Input: part model. Units: mm. Frame: model coordinates. A direction names the side the tool comes from. Coordinates: 2 decimals unless noted, no trailing zeros. Order: outer loops, then holes, each group sorted by start corner. A loop starts at its lowest first (then second) coordinate and runs counter-clockwise, first axis right, second up.
from build123d import *

# Parameters (mm, degrees)
ESQUISSE1_R             = 26.25
BOSS_EXTRU_1_DEPTH      = 5
ESQUISSE2_R             = 1.5
ENL_V_MAT_EXTRU_1_DEPTH = 5
ENL_V_START             = -5
ESQUISSE3_R             = 26.25
ESQUISSE3_R_2           = 2
ENL_V_MAT_EXTRU_2_DEPTH = 5
CONG_1_R                = 2
ESQUISSE4_R             = 1.125
ENL_V_MAT_EXTRU_3_DEPTH = 10
ESQUISSE5_R             = 4
ESQUISSE5_R_2           = 2
BOSS_EXTRU_2_DEPTH      = 3


with BuildPart() as part:
    # Esquisse1 → Boss.-Extru.1 (new body)
    with BuildSketch(Plane.XY):
        Circle(ESQUISSE1_R)
    extrude(amount=BOSS_EXTRU_1_DEPTH)

    # Esquisse2 → Enlèv. mat.-Extru.1 (cut)
    with BuildSketch(Plane.XY.offset(5)):
        Circle(ESQUISSE2_R)
    extrude(amount=-ENL_V_MAT_EXTRU_1_DEPTH, mode=Mode.SUBTRACT)

    # Esquisse3 → Enlèv. mat.-Extru.2 (cut)
    # profile 1 of 2: a face of its own
    with BuildSketch(Plane.XY.offset(5).offset(ENL_V_START)):
        Circle(ESQUISSE3_R)
        with BuildLine():
            Line((9, -2.5), (4, -2.5))
            Line((4, -2.5), (4, -19.5))
            ThreePointArc((4, -19.5), (0, -23.5), (-4, -19.5))
            Line((-4, -19.5), (-4, -2.5))
            Line((-4, -2.5), (-9, -2.5))
            ThreePointArc((-9, -2.5), (-11.5, 0), (-9, 2.5))
            Line((-9, 2.5), (-3.122498999, 2.5))
            ThreePointArc((-3.122498999, 2.5), (-2.828427125, 2.828427125), (-2.5, 3.122498999))
            Line((-2.5, 3.122498999), (-2.5, 9))
            ThreePointArc((-2.5, 9), (0, 11.5), (2.5, 9))
            Line((2.5, 9), (2.5, 3.122498999))
            ThreePointArc((2.5, 3.122498999), (2.828427125, 2.828427125), (3.122498999, 2.5))
            Line((3.122498999, 2.5), (9, 2.5))
            ThreePointArc((9, 2.5), (11.5, 0), (9, -2.5))
        make_face(mode=Mode.SUBTRACT)
    # profile 2 of 2: a face of its own
    with BuildSketch(Plane.XY.offset(5).offset(ENL_V_START)):
        with Locations((0, -19.5)):
            Circle(ESQUISSE3_R_2)
    extrude(amount=ENL_V_MAT_EXTRU_2_DEPTH, mode=Mode.SUBTRACT)

    # Congé1
    # the kernel refuses this fillet: 2 mm, written as the material it adds along each edge
    with BuildSketch(Plane(origin=(-4, -2.5, 0), x_dir=(0, -1, 0), z_dir=(0, 0, 1)), Plane(origin=(4, -2.5, 0), x_dir=(1, 0, 0), z_dir=(0, 0, 1))) as cong_1_piece_1:
        with BuildLine():
            CenterArc((CONG_1_R, -CONG_1_R), CONG_1_R, 90, 90)
            Line((0, -CONG_1_R), (0, 0))
            Line((0, 0), (CONG_1_R, 0))
        make_face()
    extrude(amount=5)
    with BuildSketch(Plane(origin=(-3.122498999, 2.5, 0), x_dir=(-1, 0, 0), z_dir=(0, 0, 1))) as cong_1_piece_2:
        with BuildLine():
            CenterArc((0.846127967, -2), CONG_1_R, 90, 41.409622109)
            ThreePointArc((-0.476747688, -0.5), (-0.227558946, -0.260311955), (0, 0))
            Line((0, 0), (0.846127967, 0))
        make_face()
    extrude(amount=5)
    with BuildSketch(Plane(origin=(-2.5, 3.122498999, 0), x_dir=(-0.7237350132500174, -0.6900779887780779, 0), z_dir=(0, 0, 1)), Plane(origin=(3.122498999, 2.5, 0), x_dir=(-0.6900779887780603, 0.7237350132500343, 0), z_dir=(0, 0, 1))) as cong_1_piece_3:
        with BuildLine():
            CenterArc((0.863575741, -1.992528413), CONG_1_R, 94.954095219, 41.409622109)
            Line((-0.583894286, -0.612372436), (0, 0))
            ThreePointArc((0, 0), (0.345430296, -0.014943173), (0.690860592, 0))
        make_face()
    extrude(amount=5)
    with BuildSketch(Plane(origin=(2.5, 3.122498999, 0), x_dir=(0.7237350132500171, -0.6900779887780782, 0), z_dir=(0, 0, 1))) as cong_1_piece_4:
        with BuildLine():
            CenterArc((0.863575741, 1.992528413), CONG_1_R, 223.636282672, 41.409622109)
            Line((-0.583894286, 0.612372436), (0, 0))
            ThreePointArc((0, 0), (0.345430296, 0.014943173), (0.690860592, 0))
        make_face()
    extrude(amount=5)

    # Esquisse4 → Enlèv. mat.-Extru.3 (cut)
    with BuildSketch(Plane.XY.offset(5)):
        with Locations((8, 0)):
            Circle(ESQUISSE4_R)
        with Locations((-8, 0)):
            Circle(ESQUISSE4_R)
        with Locations((0, 8)):
            Circle(ESQUISSE4_R)
    extrude(amount=-ENL_V_MAT_EXTRU_3_DEPTH, mode=Mode.SUBTRACT)

    # Esquisse5 → Boss.-Extru.2 (add)
    with BuildSketch(Plane.XY.offset(5)):
        with Locations((0, -19.5)):
            Circle(ESQUISSE5_R)
        with Locations((0, -19.5)):
            Circle(ESQUISSE5_R_2, mode=Mode.SUBTRACT)
    extrude(amount=BOSS_EXTRU_2_DEPTH)


solid = part.part
Item 1: Cut plane C-C on x = 8. Return loops of the section in (y, z) (3 decimals).
Response values:
outline: (-2.5, 0) - (-1.125, 0) - (-1.125, 5) - (-2.5, 5) - close; (1.125, 0) - (2.5, 0) - (2.5, 5) - (1.125, 5) - close
Item 2: Ray query, probe 1 along Y at (x, z) = (0, 2.6) (3 decimals); probe 2 along Y at (x, z) = (8, 3.1) (3 decimals); probe 3 along Z at (x, y) = (2, 4). Return the intervals inside material, ascending.
Response values:
probe 1: y = -23.5 to -21.5, -17.5 to -1.5, 1.5 to 6.875, 9.125 to 11.5
probe 2: y = -2.5 to -1.125, 1.125 to 2.5
probe 3: z = 0 to 5
Item 3: Access query for faces 4 (the face through (-7, 2.5, 2)), 5 (the face through (-4.57, -3.1, 2.46)), 6 (the face through (-0.24, 6.9, 2.54)), 7 (the face through (6, 2.5, 2)), 8 (the face through (8, -2.5, 2)). Directions: +Z, -Z, +X, -X, +Y, -Y. A direction counts if a zero-diameter tool reaches every point of the face in a straight line with its end or side. Return the directions, or none.
Response values:
face 4: +Z, -Z, -X, +Y
face 5: +Z, -Z, -X, -Y
face 6: +Z, -Z
face 7: +Z, -Z, +X, +Y
face 8: +Z, -Z, +X, -Y
Item 4: Pin query (flat end, axial travel): pin 1 Ø4 at (x, z) = (-8.5, 1.5) entering from +Y; pin 2 Ø1.3 at (x, y) = (8, 0) entering from +Z; pin 3 Ø3.5 at (x, y) = (0, 8) entering from +Z; pin 4 Ø2.5 at (x, z) = (-7, 2.5) entering from -Y. Return the tip coordinate at first contact, or that it passes through.
Response values:
pin 1: stops at y = 2.5
pin 2: passes through
pin 3: stops at z = 5
pin 4: stops at y = -2.52
Item 5: Cut plane B-B on z = 4.25. Return loops of the section in (x, y) (3 decimals).
Response values:
outline: (-9, -2.5) - (-6, -2.5) arc R2 cw to (-4, -4.5) - (-4, -19.5) arc R4 ccw to (4, -19.5) - (4, -4.5) arc R2 cw to (6, -2.5) - (9, -2.5) arc R2.5 ccw to (9, 2.5) - (3.969, 2.5) arc R2 cw to (2.845, 2.845) arc R2 cw to (2.5, 3.969) - (2.5, 9) arc R2.5 ccw to (-2.5, 9) - (-2.5, 3.969) arc R2 cw to (-2.845, 2.845) arc R2 cw to (-3.969, 2.5) - (-9, 2.5) arc R2.5 ccw to start; hole circle Ø2.25 at (-8, 0); hole circle Ø4 at (0, -19.5); hole circle Ø3 at (0, 0); hole circle Ø2.25 at (0, 8); hole circle Ø2.25 at (8, 0)
Item 6: Draft query along Y for faces 1 (the face through (-0.1, 11.5, 2.5)), 2 (the face through (9.073, 0.338, 2.535)), 3 (the face through (4, -12, 2)). Return one class per face: pulls with the +Y half, pulls with the -Y half, needs draft (parallel to the pull), parting line crosses it, or undercut.
Response values:
face 1: pulls with the +Y half
face 2: undercut
face 3: needs draft
Item 7: Cut plane A-A on y = 0. Return loops of the section in (x, z) (3 decimals), then the cut area to 3 significant figures.
Response values:
outline: (-11.5, 0) - (-9.125, 0) - (-9.125, 5) - (-11.5, 5) - close; (-6.875, 0) - (-1.5, 0) - (-1.5, 5) - (-6.875, 5) - close; (1.5, 0) - (6.875, 0) - (6.875, 5) - (1.5, 5) - close; (9.125, 0) - (11.5, 0) - (11.5, 5) - (9.125, 5) - close
area: 77.5 mm2
